from build123d import *

# Parameters (mm, degrees)
F0_W     = 38
F0_H     = 70
F1_DEPTH = 9.5
F2_W     = 19
F2_H     = 25
F3_DEPTH = 19
F4_R     = 5
F5_DEPTH = 38
F6_SIZE  = 2
F8_D     = 8.5
F8_DEPTH = 19.5
F8_TIP   = 2.5536576309


with BuildPart() as f1:
    # F0 (on Front) → F1 (new body, symmetric)
    with BuildSketch(Plane.XZ):
        Rectangle(F0_W, F0_H)
    extrude(amount=F1_DEPTH, both=True)

    # F2 (on face) → F3 (cut)
    with BuildSketch(Plane.XZ.offset(9.5)):
        with Locations((0, 22.5)):
            Rectangle(F2_W, F2_H)
    extrude(amount=-F3_DEPTH, mode=Mode.SUBTRACT)

    # F4 (on face) → F5 (cut)
    with BuildSketch(Plane.YZ.offset(19)):
        with Locations((0, 25)):
            Circle(F4_R)
    extrude(amount=-F5_DEPTH, mode=Mode.SUBTRACT)

    # F6
    f6_edges = [f1.edges().sort_by_distance(p)[0] for p in [
        (14.25, 9.5, 35),
        (-14.25, 9.5, 35),
        (-14.25, -9.5, 35),
        (14.25, -9.5, 35),
    ]]
    chamfer(f6_edges, length=F6_SIZE)

    # F8
    with Locations(Plane(origin=(0, 0, -35), x_dir=(1, 0, 0), z_dir=(0, 0, -1))):
        with Locations((-11.5, 0), (11.5, 0)):
            Hole(F8_D / 2, depth=F8_DEPTH)
            with Locations((0, 0, -(F8_DEPTH + F8_TIP / 2))):  # 118° drill point
                Cone(0, F8_D / 2, F8_TIP, mode=Mode.SUBTRACT)


solid = f1.part
Model file for the job. Use its own axes, mm. A direction names the side the tool comes from. Give positions to 0.01 mm unless a question says otherwise; leave off trailing zeros. Loops run counter-clockwise (first coordinate to the right, second up) from the corner with the lowest first, then second, coordinate; pieces in that order, holes last.
Item 1: Drill centre lines: line 1 along X through (y, z) = (-3.25, -20.5); line 2 along X through (y, z) = (3, -21); line 3 along X through (y, z) = (2.75, 32.5). Where is each one in solid material? Low to high.
Check values:
line 1: x = -19 to -14.24, -8.76 to 8.76, 14.24 to 19
line 2: x = -19 to -14.51, -8.49 to 8.49, 14.51 to 19
line 3: x = -19 to -9.5, 9.5 to 19
Item 2: Slice it at B-B (y = -1.5). Give the number of separate pieces and of enclosed holes in the cut face, plus the area to 3 significant figures.
Check values:
separate pieces: 3
enclosed holes: 0
area: 1,680 mm2
Item 3: Which spindle directions (+Z, -Z, +X, -X, +Y, -Y) get a long thin tool onto all of the face, cutting with end or side? Do faces 5 (the face through (14.32, -1.08, 20.12)), 6 (the face through (-13.785, -3.584, -25.114)). Say none if no direction does.
Check values:
face 5: +X, -X
face 6: -Z
Item 4: Slice it at A-A (x = -3.5). Write the cut outline in (y, z).
Check values:
outline: (-9.5, -35) - (9.5, -35) - (9.5, 10) - (-9.5, 10) - close
Item 5: Mould opens along X. For faces 1 (the face through (-9.5, -0.1, 19.5)), 2 (the face through (0, 0, 10)), 3 (the face through (0, 0, -35)), 4 (the face through (-19, 0, 0)) say: +X half, -X half, draft (parallel to the pull), parting line (faces both ways), or undercut.
Check values:
face 1: undercut
face 2: undercut
face 3: draft
face 4: -X half
Item 6: Drop flat-ended pins along their axis: P1, Ø6, axis at y = 0, z = 25, coming from the -X side; P2, Ø9.5, axis at x = 3, y = -3.5, coming from the +Z side; P3, Ø7.5, axis at x = 11.5, y = 0, coming from the -Z side. Give the stop position or say it passes through.
Check values:
P1: passes through
P2: stops at z = 10
P3: stops at z = -15.2
